Check sheet for the modelled part. Datum: model origin and axes. Units: mm. Give positions to 0.01 mm unless a question says otherwise; leave off trailing zeros. Order: outer loops, then holes, each group sorted by start corner. A loop starts at its lowest first (then second) coordinate and runs counter-clockwise, first axis right, second up.
```python
from build123d import *

# Parameters (mm, degrees)
SKETCH1_W           = 5.1
SKETCH1_H           = 5.1
BOSS_EXTRUDE1_DEPTH = 3
SKETCH2_R           = 26.5
SKETCH2_R_2         = 1.5
CUT_EXTRUDE1_DEPTH  = 3
FILLET1_R           = 15
SKETCH7_W           = 4.1
SKETCH7_H           = 3.1
SKETCH7_W_2         = 4.2
SKETCH7_W_3         = 5.1
SKETCH7_W_4         = 10.1
CUT_EXTRUDE4_DEPTH  = 10
CHAMFER1_SIZE       = 3
CHAMFER1_SIZE2      = 1.732050808
CUT_EXTRUDE5_DEPTH  = 10
SKETCH9_R           = 1
SKETCH9_R_2         = 1.5
CUT_EXTRUDE6_DEPTH  = 10
FILLET3_R           = 2


with BuildPart() as part:
    # Sketch1 → Boss-Extrude1 (new body)
    with BuildSketch(Plane(origin=(0, 0, 0), x_dir=(1, 0, 0), z_dir=(0, 1, 0))):
        Polygon((75, 95), (75, 110), (-75, 110), (-75, 95), (-84, 27), (-57.5, 27), (-57.5, 19.1), (-57.5, 14), (-57.5, 0), (57.5, 0), (57.5, 14), (57.5, 19.1), (57.5, 27), (84, 27), align=None)
        with Locations((52.45, 16.55)):
            Rectangle(SKETCH1_W, SKETCH1_H, mode=Mode.SUBTRACT)
        with Locations((52.45, 36.55)):
            Rectangle(SKETCH1_W, SKETCH1_H, mode=Mode.SUBTRACT)
        with Locations((-52.45, 16.55)):
            Rectangle(SKETCH1_W, SKETCH1_H, mode=Mode.SUBTRACT)
        with Locations((-52.45, 36.55)):
            Rectangle(SKETCH1_W, SKETCH1_H, mode=Mode.SUBTRACT)
    extrude(amount=BOSS_EXTRUDE1_DEPTH)

    # Sketch2 → Cut-Extrude1 (cut)
    with BuildSketch(Plane(origin=(0, 3, 0), x_dir=(1, 0, 0), z_dir=(0, 1, 0))):
        with Locations(Location((0, 53, 0), (0, 0, 270))):
            Circle(SKETCH2_R)
        with Locations(Location((23.511300474, 76.511300474, 0), (0, 0, 270))):
            Circle(SKETCH2_R_2)
        with Locations(Location((-23.511300474, 76.511300474, 0), (0, 0, 270))):
            Circle(SKETCH2_R_2)
        with Locations(Location((-23.511300474, 29.488699526, 0), (0, 0, 270))):
            Circle(SKETCH2_R_2)
        with Locations(Location((23.511300474, 29.488699526, 0), (0, 0, 270))):
            Circle(SKETCH2_R_2)
    extrude(amount=-CUT_EXTRUDE1_DEPTH, mode=Mode.SUBTRACT)

    # Fillet1
    fillet1_edges = [part.edges().sort_by_distance(p)[0] for p in [
        (-84, 1.5, -27),
        (84, 1.5, -27),
    ]]
    fillet(fillet1_edges, radius=FILLET1_R)

    # Sketch7 → Cut-Extrude4 (cut)
    with BuildSketch(Plane.XZ):
        with Locations((-14, -3.95)):
            Rectangle(SKETCH7_W, SKETCH7_H)
        with Locations((16, -19.15)):
            Rectangle(SKETCH7_W_2, SKETCH7_H)
        with Locations((-23.5, -11.55)):
            Rectangle(SKETCH7_W_3, SKETCH7_H)
        with Locations((23.5, -11.55)):
            Rectangle(SKETCH7_W_3, SKETCH7_H)
        with Locations((0, -11.55)):
            Rectangle(SKETCH7_W_4, SKETCH7_H)
    extrude(amount=-CUT_EXTRUDE4_DEPTH, mode=Mode.SUBTRACT)

    # Chamfer1
    chamfer1_edges = [part.edges().sort_by_distance(p)[0] for p in [
        (0, 0, -110),
    ]]
    chamfer1_side = [part.faces().sort_by_distance(p)[0] for p in [
        (76.421351958, 0, -69.225215197),
    ]]
    chamfer(chamfer1_edges, length=CHAMFER1_SIZE, length2=CHAMFER1_SIZE2, reference=chamfer1_side[0])

    # Sketch4 → Cut-Extrude5 (cut)
    with BuildSketch(Plane(origin=(0, 3, 0), x_dir=(1, 0, 0), z_dir=(0, 1, 0))):
        with BuildLine():
            Line((50.4, 39.1), (49.9, 39.1))
            Line((49.9, 39.1), (49.9, 38.6))
            ThreePointArc((49.9, 38.6), (49.546446609, 39.453553391), (50.4, 39.1))
        make_face()
        with BuildLine():
            ThreePointArc((54.5, 39.1), (55.353553391, 39.453553391), (55, 38.6))
            Line((55, 38.6), (55, 39.1))
            Line((55, 39.1), (54.5, 39.1))
        make_face()
        with BuildLine():
            ThreePointArc((55, 34.5), (55.353553391, 33.646446609), (54.5, 34))
            Line((54.5, 34), (55, 34))
            Line((55, 34), (55, 34.5))
        make_face()
        with BuildLine():
            Line((49.9, 34.5), (49.9, 34))
            Line((49.9, 34), (50.4, 34))
            ThreePointArc((50.4, 34), (49.546446609, 33.646446609), (49.9, 34.5))
        make_face()
        with BuildLine():
            Line((49.9, 19.1), (49.9, 18.6))
            ThreePointArc((49.9, 18.6), (49.546446609, 19.453553391), (50.4, 19.1))
            Line((50.4, 19.1), (49.9, 19.1))
        make_face()
        with BuildLine():
            ThreePointArc((49.9, 14.5), (49.546446609, 13.646446609), (50.4, 14))
            Line((50.4, 14), (49.9, 14))
            Line((49.9, 14), (49.9, 14.5))
        make_face()
        with BuildLine():
            ThreePointArc((13.9, 20.7), (14.4, 21.2), (14.9, 20.7))
            Line((14.9, 20.7), (13.9, 20.7))
        make_face()
        with BuildLine():
            ThreePointArc((18.1, 20.7), (17.6, 21.2), (17.1, 20.7))
            Line((17.1, 20.7), (18.1, 20.7))
        make_face()
        with BuildLine():
            ThreePointArc((18.1, 17.6), (17.6, 17.1), (17.1, 17.6))
            Line((17.1, 17.6), (18.1, 17.6))
        make_face()
        with BuildLine():
            ThreePointArc((13.9, 17.6), (14.4, 17.1), (14.9, 17.6))
            Line((14.9, 17.6), (13.9, 17.6))
        make_face()
        with BuildLine():
            ThreePointArc((20.95, 13.1), (21.45, 13.6), (21.95, 13.1))
            Line((21.95, 13.1), (20.95, 13.1))
        make_face()
        with BuildLine():
            ThreePointArc((26.05, 13.1), (25.55, 13.6), (25.05, 13.1))
            Line((25.05, 13.1), (26.05, 13.1))
        make_face()
        with BuildLine():
            ThreePointArc((26.05, 10), (25.55, 9.5), (25.05, 10))
            Line((25.05, 10), (26.05, 10))
        make_face()
        with BuildLine():
            ThreePointArc((20.95, 10), (21.45, 9.5), (21.95, 10))
            Line((21.95, 10), (20.95, 10))
        make_face()
        with BuildLine():
            ThreePointArc((5.05, 13.1), (4.55, 13.6), (4.05, 13.1))
            Line((4.05, 13.1), (5.05, 13.1))
        make_face()
        with BuildLine():
            ThreePointArc((5.05, 10), (4.55, 9.5), (4.05, 10))
            Line((4.05, 10), (5.05, 10))
        make_face()
        with BuildLine():
            ThreePointArc((-5.05, 13.1), (-4.55, 13.6), (-4.05, 13.1))
            Line((-4.05, 13.1), (-5.05, 13.1))
        make_face()
        with BuildLine():
            ThreePointArc((-5.05, 10), (-4.55, 9.5), (-4.05, 10))
            Line((-4.05, 10), (-5.05, 10))
        make_face()
        with BuildLine():
            ThreePointArc((-11.95, 5.5), (-12.45, 6), (-12.95, 5.5))
            Line((-12.95, 5.5), (-11.95, 5.5))
        make_face()
        with BuildLine():
            ThreePointArc((-11.95, 2.4), (-12.45, 1.9), (-12.95, 2.4))
            Line((-12.95, 2.4), (-11.95, 2.4))
        make_face()
        with BuildLine():
            ThreePointArc((-16.05, 2.4), (-15.55, 1.9), (-15.05, 2.4))
            Line((-15.05, 2.4), (-16.05, 2.4))
        make_face()
        with BuildLine():
            ThreePointArc((-16.05, 5.5), (-15.55, 6), (-15.05, 5.5))
            Line((-15.05, 5.5), (-16.05, 5.5))
        make_face()
        with BuildLine():
            ThreePointArc((-20.95, 10), (-21.45, 9.5), (-21.95, 10))
            Line((-21.95, 10), (-20.95, 10))
        make_face()
        with BuildLine():
            ThreePointArc((-20.95, 13.1), (-21.45, 13.6), (-21.95, 13.1))
            Line((-21.95, 13.1), (-20.95, 13.1))
        make_face()
        with BuildLine():
            ThreePointArc((-26.05, 13.1), (-25.55, 13.6), (-25.05, 13.1))
            Line((-25.05, 13.1), (-26.05, 13.1))
        make_face()
        with BuildLine():
            ThreePointArc((-26.05, 10), (-25.55, 9.5), (-25.05, 10))
            Line((-25.05, 10), (-26.05, 10))
        make_face()
        with BuildLine():
            Line((-49.9, 19.1), (-49.9, 18.6))
            ThreePointArc((-49.9, 18.6), (-49.546446609, 19.453553391), (-50.4, 19.1))
            Line((-50.4, 19.1), (-49.9, 19.1))
        make_face()
        with BuildLine():
            ThreePointArc((-49.9, 14.5), (-49.546446609, 13.646446609), (-50.4, 14))
            Line((-50.4, 14), (-49.9, 14))
            Line((-49.9, 14), (-49.9, 14.5))
        make_face()
        with BuildLine():
            ThreePointArc((-50.4, 39.1), (-49.546446609, 39.453553391), (-49.9, 38.6))
            Line((-49.9, 38.6), (-49.9, 39.1))
            Line((-49.9, 39.1), (-50.4, 39.1))
        make_face()
        with BuildLine():
            Line((-49.9, 34), (-50.4, 34))
            ThreePointArc((-50.4, 34), (-49.546446609, 33.646446609), (-49.9, 34.5))
            Line((-49.9, 34.5), (-49.9, 34))
        make_face()
        with BuildLine():
            ThreePointArc((-54.5, 39.1), (-55.353553391, 39.453553391), (-55, 38.6))
            Line((-55, 38.6), (-55, 39.1))
            Line((-55, 39.1), (-54.5, 39.1))
        make_face()
        with BuildLine():
            ThreePointArc((-55, 34.5), (-55.353553391, 33.646446609), (-54.5, 34))
            Line((-54.5, 34), (-55, 34))
            Line((-55, 34), (-55, 34.5))
        make_face()
    extrude(amount=-CUT_EXTRUDE5_DEPTH, mode=Mode.SUBTRACT)

    # Sketch9 → Cut-Extrude6 (cut)
    with BuildSketch(Plane(origin=(0, 3, 0), x_dir=(1, 0, 0), z_dir=(0, 1, 0))):
        with Locations(Location((52.45, 26.5, 0), (0, 0, 270))):
            Circle(SKETCH9_R)
        with Locations(Location((52.45, 8, 0), (0, 0, 270))):
            Circle(SKETCH9_R)
        with Locations(Location((67, 100, 0), (0, 0, 270))):
            Circle(SKETCH9_R_2)
        with Locations(Location((68.915529111, 80, 0), (0, 0, 270))):
            Circle(SKETCH9_R_2)
        with Locations(Location((-52.45, 8, 0), (0, 0, 90))):
            Circle(SKETCH9_R)
        with Locations(Location((-52.45, 26.5, 0), (0, 0, 90))):
            Circle(SKETCH9_R)
        with Locations(Location((-68.915529111, 80, 0), (0, 0, 90))):
            Circle(SKETCH9_R_2)
        with Locations(Location((-67, 100, 0), (0, 0, 90))):
            Circle(SKETCH9_R_2)
    extrude(amount=-CUT_EXTRUDE6_DEPTH, mode=Mode.SUBTRACT)

    # Fillet3
    fillet3_edges = [part.edges().sort_by_distance(p)[0] for p in [
        (57.5, 1.5, 0),
        (-57.5, 1.5, 0),
        (-57.5, 1.5, -27),
        (57.5, 1.5, -27),
    ]]
    fillet(fillet3_edges, radius=FILLET3_R)


solid = part.part
```
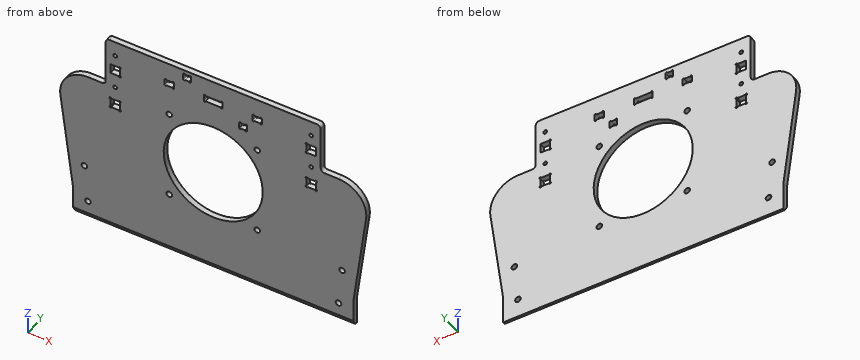
(1) Cross-section at C-C on z = -48. Enter the section's corners in (x, y).
Response values:
outline: (-81.22, 0) - (-26.02, 0) - (-26.02, 3) - (-81.22, 3) - close; (26.02, 0) - (81.22, 0) - (81.22, 3) - (26.02, 3) - close
(2) Material ranges on L1, parallel to X at y = 1.15, z = -8; L2, parallel to X at y = 2.7, z = -15.5; L3, parallel to Z at x = 17.5, y = 1.8, recorded low to high.
Response values:
L1: x = -57.5 to -53.45, -51.45 to 51.45, 53.45 to 57.5
L2: x = -57.5 to -55, -49.9 to 49.9, 55 to 57.5
L3: z = -110 to -72.9, -33.1 to -21.19, -17.11 to 0
(3) Cross-section at B-B on y = 0.5. Count the separate pieces of the cut face and the enclosed holes in it, then the cut area to 3 significant figures.
Response values:
separate pieces: 1
enclosed holes: 22
area: 13,200 mm2
(4) Gauge pin test, flat ends, axial feed: pin 1 Ø0.9 at (y, z) = (1, -11.5) entering from -X; pin 2 Ø1.2 at (x, z) = (55, -39.1) entering from -Y; pin 3 Ø1 at (y, z) = (0.5, -54.5) entering from +X; pin 4 Ø0.7 at (x, y) = (16, 1) entering from -Z. Record the tip position at first contact, or that the pin passes through.
Response values:
pin 1: stops at x = -57.5
pin 2: stops at y = 0
pin 3: stops at x = 80.43
pin 4: stops at z = -109.34
(5) Cross-section at A-A on z = -73. Enter the section's corners in (x, y), then the cut area to 3 significant figures.
Response values:
outline: (-77.91, 0) - (-17.39, 0) - (-17.39, 3) - (-77.91, 3) - close; (17.39, 0) - (77.91, 0) - (77.91, 3) - (17.39, 3) - close
area: 363 mm2
